Read the model definition and answer for the solid it produces. Units are mm, in the model's axes. A direction names the side the tool comes from. Coordinates: 2 decimals unless noted, no trailing zeros. Write each loop counter-clockwise with the first axis right and the second up, starting at its lowest first coordinate (ties: lowest second). Pieces come first, ordered by that corner, then holes.
1) Each of these flat-tipped pins is pushed along its axis until it touches: pin 1 Ø3 at (y, z) = (7.5, 89) entering from +X; pin 2 Ø5 at (x, y) = (-6, 6) entering from +Z. Where does it stop, or does it pass through?
2) The part is cut by section D-D (y = 5). Give the number of separate pieces and of enclosed holes in the cut face, then the cut area to 3 significant figures.
3) The part is cut by section C-C (x = 0). Determine the outline of the cut face in (y, z), then the cut area to 3 significant figures.
4) The part is cut by section B-B (z = 0). Determine the outline of the cut face in (x, y), then the cut area to 3 significant figures.
5) Find the intervals of material crossed by line 1 (Y direction, x = 95, z = 97); line 2 (X direction, y = 5.25, z = -68); line 3 (X direction, y = 3.25, z = -46.5), in increasing order.
6) Determine the mould class of faces 5 (the face through (-58, 5, 100)), 6 (the face through (97, 3, -85)), 7 (the face through (-97.5, 5.1, 1.2)) for opening direction Z: +Z half, -Z half, draft (parallel to the pull), parting line (faces both ways), or undercut.
7) Which of the six approach directions +Z, -Z, +X, -X, +Y, -Y give full straight-line access (tool end or side, diameter ignored) to faces 1 (the face through (93, 3, 85)), 2 (the face through (-90, 5, 90)), 3 (the face through (-15, 5, 75)), 4 (the face through (100, 5, 98))?
8) The part is cut by section A-A (x = -95). Determine the outline of the cut face in (y, z), then the cut area to 3 significant figures.
from build123d import *

# Parameters (mm, degrees)
ESQUISSE1_R             = 15
BASE_DEPTH              = 10
ESQUISSE2_R             = 2.5
ENL_V_MAT_EXTRU_1_DEPTH = 224.830292856


with BuildPart() as part:
    # Esquisse1 → BASE (new body)
    with BuildSketch(Plane(origin=(0, 0, 0), x_dir=(1, 0, 0), z_dir=(0, 1, 0))):
        Polygon((-100, 95), (-90, 95), (-90, 85), (-100, 85), (-100, -85), (-90, -85), (-90, -95), (-100, -95), (-100, -100), (-15, -100), (-15, -50), (15, -50), (15, -100), (100, -100), (100, -95), (90, -95), (90, -85), (100, -85), (100, 85), (90, 85), (90, 95), (100, 95), (100, 100), (-100, 100), align=None)
        with Locations(Location((0, 0, 0), (0, 0, 270))):
            Circle(ESQUISSE1_R, mode=Mode.SUBTRACT)
    extrude(amount=BASE_DEPTH)

    # Esquisse2 → Enlèv. mat.-Extru.1 (cut, through all)
    with BuildSketch(Plane.XY.offset(100)):
        with Locations((-95, 5)):
            Circle(ESQUISSE2_R)
        with Locations(Location((95, 5, 0), (0, 0, 180))):
            Circle(ESQUISSE2_R)
    extrude(amount=-ENL_V_MAT_EXTRU_1_DEPTH, mode=Mode.SUBTRACT)


solid = part.part
Reported:
1. pin 1: stops at x = 90
1. pin 2: stops at z = 50
2. separate pieces: 7
2. enclosed holes: 1
2. area: 35,600 mm2
3. outline: (0, -100) - (10, -100) - (10, -15) - (0, -15) - close; (0, 15) - (10, 15) - (10, 50) - (0, 50) - close
3. area: 1,200 mm2
4. outline: (-100, 0) - (-15, 0) - (-15, 10) - (-100, 10) - close; (15, 0) - (100, 0) - (100, 10) - (15, 10) - close; hole circle Ø5 at (-95, 5); hole circle Ø5 at (95, 5)
4. area: 1,660 mm2
5. line 1: y = 0 to 2.5, 7.5 to 10
5. line 2: x = -100 to -97.49, -92.51 to 92.51, 97.49 to 100
5. line 3: x = -100 to -96.79, -93.21 to 93.21, 96.79 to 100
6. face 5: +Z half
6. face 6: undercut
6. face 7: draft
7. face 1: +X, +Y, -Y
7. face 2: -X, +Y, -Y
7. face 3: +Z, +Y, -Y
7. face 4: +Z, -Z, +X, +Y, -Y
8. outline: (0, -100) - (2.5, -100) - (2.5, -95) - (0, -95) - close; (0, -85) - (2.5, -85) - (2.5, 85) - (0, 85) - close; (0, 95) - (2.5, 95) - (2.5, 100) - (0, 100) - close; (7.5, -100) - (10, -100) - (10, -95) - (7.5, -95) - close; (7.5, -85) - (10, -85) - (10, 85) - (7.5, 85) - close; (7.5, 95) - (10, 95) - (10, 100) - (7.5, 100) - close
8. area: 900 mm2
